```python
from build123d import *

# Parameters (mm, degrees)
F0_R     = 2.4
F0_R_2   = 5
F1_DEPTH = 6


with BuildPart() as f1:
    # F0 (on Front) → F1 (new body)
    with BuildSketch(Plane.XZ):
        with BuildLine():
            add(Edge.make_bspline(
                [(-4.5759957999, -5.3663848974), (-3.3944030614, -5.0263522526), (-1.1564816937, -4.5735976346), (1.1915972707, -5.7397107149), (2.3027864337, -6.4089476665)],
                knots=[0, 0, 0, 0, 0.4673689741, 0.8842484986, 0.8842484986, 0.8842484986, 0.8842484986], degree=3))
            add(Edge.make_bspline(
                [(2.3027864337, -6.4089476665), (2.6113211695, -6.5947691746), (2.9201786156, -6.7898015167), (3.2289242512, -6.9888996834)],
                knots=[0.8842484986, 0.8842484986, 0.8842484986, 0.8842484986, 1, 1, 1, 1], degree=3))
            ThreePointArc((3.2289242512, -6.9888996834), (15.001806232, 0.0655571744), (3.2289242512, 7.1200140322))
            add(Edge.make_bspline(
                [(2.1087657664, 6.3947083815), (2.4816893958, 6.631967091), (2.8553011873, 6.8792507811), (3.2289242512, 7.1200140322)],
                knots=[0.8599364178, 0.8599364178, 0.8599364178, 0.8599364178, 1, 1, 1, 1], degree=3))
            add(Edge.make_bspline(
                [(-4.5759957999, 5.628613595), (-3.3951999873, 5.2883114962), (-1.214946794, 4.4452120066), (1.0628103891, 5.729258398), (2.1087657664, 6.3947083815)],
                knots=[0, 0, 0, 0, 0.4670939015, 0.8599364178, 0.8599364178, 0.8599364178, 0.8599364178], degree=3))
            ThreePointArc((-4.5759957999, 5.628613595), (-13.022586423, 0.1311143488), (-4.5759957999, -5.3663848974))
        make_face()
        with Locations((-7.0102557888, 0.1311143488)):
            Circle(F0_R, mode=Mode.SUBTRACT)
        with Locations((7.001806232, 0.0655571744)):
            Circle(F0_R_2, mode=Mode.SUBTRACT)
    extrude(amount=F1_DEPTH)


solid = f1.part
```
The model under review builds one solid part; all positions refer to its coordinate system, in mm. Coordinates: 2 decimals unless noted, no trailing zeros. Write each loop counter-clockwise with the first axis right and the second up, starting at its lowest first coordinate (ties: lowest second). Pieces come first, ordered by that corner, then holes. Notation, with made-up numbers: (73, 20) - (80, 20) arc R15 cw to (80, 39) - close; hole circle Ø4 at (68, 47). An arc over 180 degrees is marked (long way). Answer in a Markdown table with one row per item. Add a question column.
Q1. Consider section B-B on x = -7.25. Give the boundary of the cut face in (y, z).
Q2. Consider section A-A on z = 1. Give the boundary of the cut face in (x, y), then the cut area to 4 significant figures.
Q3. Consider section D-D on z = -0.75. Give the boundary of the cut face in (x, y).
Q4. To check wall thickness, follow line 1 along X through (y, z) = (-4.5, -1.5); line 2 along X through (y, z) = (-4.25, 0); line 3 along Z through (x, y) = (6.75, -3.5). State the ranges of each line that lie inside material, in increasing order. Write a range as from..to.
Q5. Draft analysis for pull direction X (two halves, no side actions). For faces 1 (the face through (-8.78, -2.96, 1.75)), 2 (the face through (1, 0, 0)), 3 (the face through (15, -3, 0)), 4 (the face through (11.77, -2.96, 1.57)), state which applies: +X half, -X half, draft (parallel to the pull), parting line (faces both ways), or undercut.
Q6. Clearance check with flat-ended pins moving along their axes: pin 1 (2 mm diameter, centred on x = 0, y = -4, fed in from -Z); pin 2 (9 mm diameter, centred on x = 7, z = 0.07, fed in from -Y); pin 3 (2 mm diameter, centred on y = -5, z = -2, fed in from +X); pin 4 (2 mm diameter, centred on y = -3, z = -3.5, fed in from +X). State where each tip first meets the part, or that it passes through.
Q7. Consider section C-C on z = 3. Give the boundary of the cut face in (x, y), then the cut area to 3 significant figures.
Answers below:
| question | item | result |
|---|---|---|
| 1 | outline | (-6, -5.88) - (0, -5.88) - (0, -2.26) - (-6, -2.26) - close; (-6, 2.52) - (0, 2.52) - (0, 6.14) - (-6, 6.14) - close |
| 2 | outline | (-12.96, -6) - (-9.25, -6) - (-9.25, 0) - (-12.96, 0) - close; (-4.77, -6) - (2.09, -6) - (2.09, 0) - (-4.77, 0) - close; (11.91, -6) - (14.95, -6) - (14.95, 0) - (11.91, 0) - close |
| 2 | area | 81.65 mm² |
| 3 | outline | (-12.96, -6) - (-9.24, -6) - (-9.24, 0) - (-12.96, 0) - close; (-4.78, -6) - (2.07, -6) - (2.07, 0) - (-4.78, 0) - close; (11.93, -6) - (14.96, -6) - (14.96, 0) - (11.93, 0) - close |
| 4 | line 1 | -12.8..-8.77, -5.25..2.25, 11.75..14.85 |
| 4 | line 2 | -13.02..-9.41, -4.61..2, 12..15 |
| 4 | line 3 | -7.93..-4.93, 5.06..8.06 |
| 5 | face 1 | undercut |
| 5 | face 2 | draft |
| 5 | face 3 | parting line |
| 5 | face 4 | undercut |
| 6 | pin 1 | z = -5.69 |
| 6 | pin 2 | through |
| 6 | pin 3 | x = 14.93 |
| 6 | pin 4 | x = 14.58 |
| 7 | outline | (-12.29, -6) - (2.95, -6) - (2.95, 0) - (-12.29, 0) - close; (11.05, -6) - (14.44, -6) - (14.44, 0) - (11.05, 0) - close |
| 7 | area | 112 mm² |
